```python
from build123d import *

# Parameters (mm, degrees)
F0_R     = 3.175
F1_DEPTH = 30.48


with BuildPart() as f1:
    # F0 (on Front) → F1 (new body)
    with BuildSketch(Plane.XZ):
        with BuildLine():
            Line((9.510055, 114.833363), (9.343463, 116.150762))
            ThreePointArc((9.343463, 116.150762), (-0.334404, 123.819128), (-9.450303, 115.490543))
            ThreePointArc((-9.450303, 115.490543), (-0.596442, 104.793693), (9.525, 114.3))
            ThreePointArc((9.525, 114.3), (9.521263, 114.566786), (9.510055, 114.833363))
        make_face()
        with Locations((0, 114.3)):
            Circle(F0_R, mode=Mode.SUBTRACT)
        with BuildLine():
            ThreePointArc((9.510055, 114.833363), (9.449745, 115.494969), (9.343463, 116.150762))
            Line((9.343463, 116.150762), (9.510055, 114.833363))
        make_face()
        with BuildLine():
            ThreePointArc((9.525, 114.3), (-0.596442, 104.793693), (-9.450303, 115.490543))
            Line((-9.450303, 115.490543), (-15.735324, 65.601239))
            ThreePointArc((-15.735324, 65.601239), (0.055273, 79.374904), (15.749574, 65.491615))
            Line((15.749574, 65.491615), (9.510055, 114.833363))
            ThreePointArc((9.510055, 114.833363), (9.521263, 114.566786), (9.525, 114.3))
        make_face()
        with Locations((-3.175, 100.0252)):
            Circle(F0_R, mode=Mode.SUBTRACT)
        with BuildLine():
            Line((-15.764817, 65.367128), (-15.735324, 65.601239))
            ThreePointArc((-15.735324, 65.601239), (-15.750506, 65.484238), (-15.764817, 65.367128))
        make_face()
        with BuildLine():
            ThreePointArc((15.749574, 65.491615), (0.055273, 79.374904), (-15.735324, 65.601239))
            Line((-15.735324, 65.601239), (-15.764817, 65.367128))
            Line((-15.764817, 65.367128), (-15.12686, 58.684014))
            ThreePointArc((-15.12686, 58.684014), (1.642434, 47.710192), (15.794203, 61.90038))
            ThreePointArc((15.794203, 61.90038), (15.854788, 62.699171), (15.875, 63.5))
            ThreePointArc((15.875, 63.5), (15.843612, 64.49778), (15.749574, 65.491615))
        make_face()
        with Locations((0, 63.5)):
            Circle(F0_R, mode=Mode.SUBTRACT)
        with BuildLine():
            Line((-15.12686, 58.684014), (-15.764817, 65.367128))
            ThreePointArc((-15.764817, 65.367128), (-15.803162, 61.991461), (-15.12686, 58.684014))
        make_face()
        with BuildLine():
            ThreePointArc((15.794203, 61.90038), (1.642434, 47.710192), (-15.12686, 58.684014))
            Line((-15.12686, 58.684014), (-9.525, 0))
            ThreePointArc((-9.525, 0), (0, 9.525), (9.525, 0))
            ThreePointArc((9.525, 0), (6.97061, -6.491242), (0.677501, -9.500875))
            Line((0.677501, -9.500875), (44.732484, -7.932102))
            ThreePointArc((44.732484, -7.932102), (36.513087, -0.09504), (44.541716, 7.937341))
            Line((44.541716, 7.937341), (18.932946, 8.853652))
            ThreePointArc((18.932946, 8.853652), (13.224775, 11.574196), (11.307494, 17.599858))
            Line((11.307494, 17.599858), (15.794203, 61.90038))
        make_face()
        with BuildLine():
            ThreePointArc((9.525, 0), (0, 9.525), (-9.525, 0))
            ThreePointArc((-9.525, 0), (-6.735192, -6.735192), (0, -9.525))
            Line((0, -9.525), (0.677501, -9.500875))
            ThreePointArc((0.677501, -9.500875), (6.97061, -6.491242), (9.525, 0))
        make_face()
        Circle(F0_R, mode=Mode.SUBTRACT)
        with BuildLine():
            Line((0.677501, -9.500875), (0, -9.525))
            ThreePointArc((0, -9.525), (0.338965, -9.518967), (0.677501, -9.500875))
        make_face()
        with BuildLine():
            ThreePointArc((52.387513, 0.00037), (50.095002, 5.580514), (44.541716, 7.937341))
            ThreePointArc((44.541716, 7.937341), (36.513087, -0.09504), (44.732484, -7.932102))
            ThreePointArc((44.732484, -7.932102), (50.161669, -5.511516), (52.387513, 0.00037))
        make_face()
        with Locations((44.450013, 0.00037)):
            Circle(F0_R, mode=Mode.SUBTRACT)
    extrude(amount=F1_DEPTH)


solid = f1.part
```
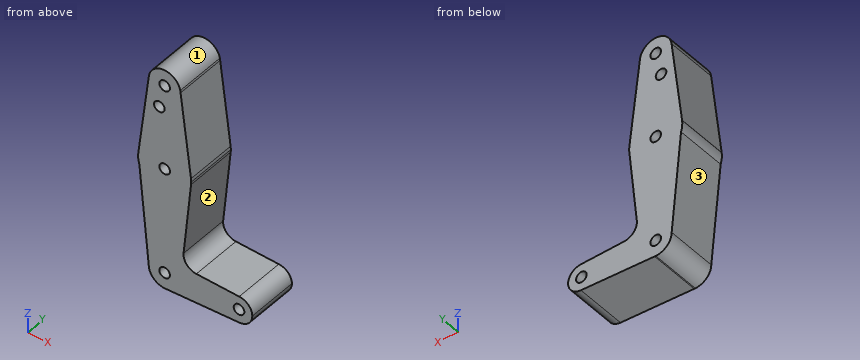
Model file for the job. Use its own axes, mm. Face numbers are marked on the shaded views. Coordinates: 2 decimals unless noted, no trailing zeros. Loops run counter-clockwise (first coordinate to the right, second up) from the corner with the lowest first, then second, coordinate; pieces in that order, holes last. Notation, with made-up numbers: (55, -33.5) - (98, -33.5) arc R11 ccw to (98, -29.5) - close; hole circle Ø3 at (69.25, 29.5). An arc over 180 degrees is marked (long way). Answer as a JSON object with one key per item and string values. Group by question number.
(1) Cut at B-B (z = 105). Give the cut face in (x, y).
(2) Cut at A-A (y = -16). State how many separate pieces and enclosed holes the cut face has, then the cut area to 3 significant figures.
(3) Cut at C-C (x = 39). Give the cut face in (y, z).
(4) Two-plate mould, pull along Z, no slides. Class the marked faces 1, 2 and 3: released by +Z, released by -Z, zero draft, split by the parting line, or undercut.
(5) Flat gauge pins, fed straight in: pin 1 (6 mm diameter, centred on y = -12.5, z = 48.5, fed in from +X); pin 2 (10 mm diameter, centred on x = 24, y = -5.5, fed in from -Z); pin 3 (5 mm diameter, centred on x = 0, z = 0, fed in from -Y); pin 4 (10 mm diameter, centred on y = -25.5, z = 74, fed in from +X). Where does each tip first touch, or does it go through?
(6) Probe line 1 along X through (y, z) = (-20, 114); line 2 along X through (y, z) = (-24.5, 102); line 3 along X through (y, z) = (-24, 43.5). List the from-to ranges inside material, lowest first.
Geometry says:
{
 "1": {"outline": "(-10.77, -30.48) - (10.75, -30.48) - (10.75, 0) - (-10.77, 0) - close"},
 "2": {"separate pieces": "1", "enclosed holes": "5", "area": "3,760 mm^2"},
 "3": {"outline": "(-30.48, -8.14) - (0, -8.14) - (0, 8.14) - (-30.48, 8.14) - close"},
 "4": {"face 1": "released by +Z", "face 2": "undercut", "face 3": "released by -Z"},
 "5": {"pin 1": "stops at x = 14.74", "pin 2": "stops at z = -8.85", "pin 3": "passes through", "pin 4": "stops at x = 15.31"},
 "6": {"line 1": "x = -9.64 to -3.16, 3.16 to 9.62", "line 2": "x = -11.15 to -5.66, -0.69 to 11.13", "line 3": "x = -13.68 to 13.93"}
}
